from build123d import *

# Parameters (mm, degrees)
SKETCH_1_W           = 20
SKETCH_1_H           = 20
EXTRUDE_1_DEPTH      = 4
SKETCH_2_R           = 1.6
CUT_EXTRUDE_1_DEPTH  = 4
SKETCH_3_R           = 1.6
CUT_EXTRUDE_2_DEPTH  = 4
EXTRUDE_2_DEPTH      = 50
SKETCH_6_R           = 1.6
CUT_EXTRUDE_3_DEPTH  = 4
SKETCH_7_W           = 10
SKETCH_7_H           = 4
EXTRUDE_3_DEPTH      = 40
EXTRUDE_3_DEPTH_BACK = 20
SKETCH_8_R           = 1.6
CUT_EXTRUDE_4_DEPTH  = 40


with BuildPart() as part:
    # ｽｹｯﾁ1 → ﾎﾞｽ - 押し出し1 (new body)
    with BuildSketch(Plane.XY):
        Polygon((-10.994705775, -41.083316507), (-50.994705775, -1.013434561), (-43.9174693, 6.051459201), (-3.987925088, -33.948540799), align=None)
        with Locations((-0.994705775, -43.948540799)):
            Rectangle(SKETCH_1_W, SKETCH_1_H)
    extrude(amount=EXTRUDE_1_DEPTH)

    # ｽｹｯﾁ2 → ｶｯﾄ - 押し出し1 (cut)
    with BuildSketch(Plane.XY.offset(4)):
        with Locations((-5.994705775, -38.948540799)):
            Circle(SKETCH_2_R)
        with Locations((-0.994705775, -38.948540799)):
            Circle(SKETCH_2_R)
        with Locations((4.005294225, -38.948540799)):
            Circle(SKETCH_2_R)
        with Locations((-0.994705775, -48.948540799)):
            Circle(SKETCH_2_R)
        with Locations((4.005294225, -48.948540799)):
            Circle(SKETCH_2_R)
        with Locations((-5.994705775, -48.948540799)):
            Circle(SKETCH_2_R)
    extrude(amount=-CUT_EXTRUDE_1_DEPTH, mode=Mode.SUBTRACT)

    # ｽｹｯﾁ3 → ｶｯﾄ - 押し出し2 (cut)
    with BuildSketch(Plane.XY.offset(4)):
        with Locations((-40.391193775, -4.558224156)):
            Circle(SKETCH_3_R)
        with Locations((-35.391193775, -9.566959399)):
            Circle(SKETCH_3_R)
        with Locations((-30.391193775, -14.575992494)):
            Circle(SKETCH_3_R)
    extrude(amount=-CUT_EXTRUDE_2_DEPTH, mode=Mode.SUBTRACT)

    # ｽｹｯﾁ4 → ﾎﾞｽ - 押し出し2 (add)
    with BuildSketch(Plane(origin=(0, 0, 0), x_dir=(-1, 0, 0), z_dir=(0, 0, -1))):
        Polygon((43.9174693, 6.051459201), (50.994705775, -1.013434561), (48.168809817, -3.844267497), (41.091536457, 3.220539992), align=None)
    extrude(amount=EXTRUDE_2_DEPTH)

    # ｽｹｯﾁ6 → ｶｯﾄ - 押し出し3 (cut)
    with BuildSketch(Plane(origin=(-24.946130174, 24.989712277, 0), x_dir=(0.707723648, 0.706489376, 0), z_dir=(-0.706489376, 0.707723648, 0))):
        with Locations((-31.806139927, 44)):
            Circle(SKETCH_6_R)
        with Locations((-31.806139927, 37)):
            Circle(SKETCH_6_R)
        with Locations((-31.806139927, 30)):
            Circle(SKETCH_6_R)
        with Locations((-31.806139927, 23)):
            Circle(SKETCH_6_R)
        with Locations((-31.806139927, 16)):
            Circle(SKETCH_6_R)
        with Locations((-31.806139927, 9)):
            Circle(SKETCH_6_R)
        with Locations((-31.806139927, 2)):
            Circle(SKETCH_6_R)
    extrude(amount=-CUT_EXTRUDE_3_DEPTH, mode=Mode.SUBTRACT)

    # ｽｹｯﾁ7 → ﾎﾞｽ - 押し出し3 (add, two sides)
    with BuildSketch(Plane(origin=(-24.946130174, 24.989712277, 0), x_dir=(0.707723648, 0.706489376, 0), z_dir=(-0.706489376, 0.707723648, 0))) as extrude_3_sk:
        with Locations((-31.806139927, 48)):
            Rectangle(SKETCH_7_W, SKETCH_7_H)
    extrude(amount=EXTRUDE_3_DEPTH)
    extrude(extrude_3_sk.sketch, amount=-EXTRUDE_3_DEPTH_BACK)

    # ｽｹｯﾁ8 → ｶｯﾄ - 押し出し4 (cut)
    with BuildSketch(Plane.XY.offset(-46)):
        with Locations((-72.183215705, 27.289339983)):
            Circle(SKETCH_8_R)
        with Locations((-68.650768824, 23.750721746)):
            Circle(SKETCH_8_R)
        with Locations((-65.118321943, 20.212103508)):
            Circle(SKETCH_8_R)
        with Locations((-61.585875062, 16.67348527)):
            Circle(SKETCH_8_R)
        with Locations((-58.053428181, 13.134867033)):
            Circle(SKETCH_8_R)
        with Locations((-54.5209813, 9.596248795)):
            Circle(SKETCH_8_R)
        with Locations((-50.988534419, 6.057630557)):
            Circle(SKETCH_8_R)
        with Locations((-41.804172528, -3.14277686)):
            Circle(SKETCH_8_R)
        with Locations((-38.271725646, -6.681395098)):
            Circle(SKETCH_8_R)
    extrude(amount=-CUT_EXTRUDE_4_DEPTH, mode=Mode.SUBTRACT)


solid = part.part
Check sheet for the modelled part. Datum: model origin and axes. Units: mm. A direction names the side the tool comes from. Give positions to 0.01 mm unless a question says otherwise; leave off trailing zeros. Loops run counter-clockwise (first coordinate to the right, second up) from the corner with the lowest first, then second, coordinate; pieces in that order, holes last. Notation, with made-up numbers: M -28,43.25 L 15,43.25 A14 ccw 15,62.25 Z; hole C 76.5,-27 d5. An arc over 180 degrees is marked long. Use a Markdown table: item, result. Add a question column.
Q1. Sectioned sample at A-A, the plane x = -65. Record the cut outline in (y, z), then the cut area to 3 significant figures.
Q2. Sectioned sample at C-C, the plane y = -29.5. Record the cut outline in (x, z), then the cut area to 3 significant figures.
Q3. Mould release check, pull along Z, two halves, no side actions. Record for faces 1 (the flat face through (-56, 8, -50)), 2 (the cylindrical face through (-56.12, 9.67, -47.97)), 3 (the cylindrical face through (-45.45, 1.73, -31.35)): pulls with the +Z half, pulls with the -Z half, needs draft (parallel to the pull), parting line crosses it, or undercut.
Q4. Scan lines: line 1 along Y through (x, z) = (-61, -47); line 2 along Y through (x, z) = (-26.5, 2); line 3 along X through (y, z) = (-2, -14.5). Record each from-to range of solid material in increasing order. Write a range as [from, to].
Q5. Sectioned sample at B-B, the plane z = -12. Record the cut outline in (x, y).
Q6. Tool access check on faces 4 (the flat face through (-46.25, -1.93, -22.68)), 5 (the cylindrical face through (-43.403, -3.072, -47.972)), 6 (the flat face through (2, -33.949, 2)), 7 (the flat face through (-60, 18, -46)). Record the directions out of +Z, -Z, +X, -X, +Y, -Y that give a thin tool (end or side, any length) a straight path to the whole face; none if there is none.
Q7. Go/stop test with flat-tipped pins: pin 1 (5 mm diameter, centred on x = -36.5, z = -4, fed in from +Y); pin 2 (4 mm diameter, centred on x = -5.99, y = -38.95, fed in from -Z); pin 3 (17.5 mm diameter, centred on x = -67.5, y = 15.5, fed in from +Z). Record where each tip stops, or that it passes through.
Verdict:
| question | item | result |
|---|---|---|
| 1 | outline | M 13.02,-50 L 18.62,-50 L 18.62,-46 L 13.02,-46 Z; M 21.81,-50 L 27.17,-50 L 27.17,-46 L 21.81,-46 Z |
| 1 | area | 43.9 mm^2 |
| 2 | outline | M -22.56,0 L -8.43,0 L -8.43,4 L -22.56,4 Z |
| 2 | area | 56.5 mm^2 |
| 3 | face 1 | pulls with the -Z half |
| 3 | face 2 | needs draft |
| 3 | face 3 | undercut |
| 4 | line 1 | [9.01, 15.18], [18.16, 23.16] |
| 4 | line 2 | [-25.55, -11.4] |
| 4 | line 3 | [-50.01, -46.32] |
| 5 | outline | M -50.99,-1.01 L -48.17,-3.84 L -41.09,3.22 L -43.92,6.05 Z |
| 6 | face 4 | +X, -Y |
| 6 | face 5 | -Z |
| 6 | face 6 | +Z, -Z, +X, +Y |
| 6 | face 7 | +Z, -X, +Y |
| 7 | pin 1 | through |
| 7 | pin 2 | z = 0 |
| 7 | pin 3 | z = -46 |
